```python
from build123d import *

# Parameters (mm, degrees)
F0_R         = 38.1
F1_DEPTH     = 381
F2_R         = 25.4
F3_DEPTH     = 304.8
F4_W         = 38.1
F4_H         = 63.5
F5_DEPTH     = 12.7
F7_DEPTH     = 203.2
F8_R         = 38.09999
F9_T3_ANGLE  = 359.64
F9_S4_R      = 38.1
F9_T5_DEPTH  = 21
F9_T8_ANGLE  = 230.2151920397
F9_S9_R      = 38.1
F9_T10_DEPTH = 20
F10_W        = 50.8
F10_H        = 12.7
F11_DEPTH    = 25.4
F13_DEPTH    = 12.7
F15_D        = 25.4
F16_W        = 25.4
F16_H        = 12.7
F17_DEPTH    = 12.7
F19_DEPTH    = 12.7
F21_D        = 12.7


# Not quite as in the source:
# - a fillet or chamfer that OpenCascade refuses, or shapes differently, is made with other operations: its cross-section is extruded or revolved along the edge and cut away or added
# - a fillet or chamfer is up to 0.001 mm smaller than in the source, because OpenCascade refuses the exact size


with BuildPart() as f1:
    # F0 (on Top) → F1 (new body)
    with BuildSketch(Plane.XY):
        Circle(F0_R)
    extrude(amount=F1_DEPTH)

    # F2 (on Top) → F3 (join)
    with BuildSketch(Plane.XY):
        Circle(F2_R)
    extrude(amount=-F3_DEPTH)

    # F4 (on Top) → F5 (join)
    with BuildSketch(Plane.XY):
        with Locations((19.05, 31.75)):
            Rectangle(F4_W, F4_H)
        with Locations((-19.05, 31.75)):
            Rectangle(F4_W, F4_H)
    extrude(amount=F5_DEPTH)

    # F6 (on face) → F7 (join)
    with BuildSketch(Plane.XY.offset(12.7)):
        with BuildLine():
            ThreePointArc((0.6819155813, 38.0938970327), (9.2181974345, 42.0397400715), (12.7, 50.7755763829))
            ThreePointArc((12.7, 50.7755763829), (-8.7358363114, 59.9937738174), (-0.6819155813, 38.0938970327))
            ThreePointArc((-0.6819155813, 38.0938970327), (0, 38.1), (0.6819155813, 38.0938970327))
        make_face()
        with BuildLine():
            ThreePointArc((0.6819155813, 38.0938970327), (0, 38.1), (-0.6819155813, 38.0938970327))
            ThreePointArc((-0.6819155813, 38.0938970327), (0, 38.0755763829), (0.6819155813, 38.0938970327))
        make_face()
    extrude(amount=F7_DEPTH)

    # F8 (radius 38.1 in the source; OpenCascade refuses exactly that, so slightly less here)
    f8_edges = [f1.edges().sort_by_distance(p)[0] for p in [
        (-38.1, 63.5, 6.35),
        (38.1, 63.5, 6.35),
    ]]
    fillet(f8_edges, radius=F8_R)

    # F9: fillet of radius 12.7 on 2 edges, made by hand


with BuildPart() as f9_tool1:
    # F9_s2 → F9_t3 (revolve)
    with BuildSketch(Plane.XZ.offset(-50.7755763829)):
        with BuildLine():
            ThreePointArc((0, 215.9), (8.9802561211, 212.1802561211), (12.7, 203.2))
            Line((12.7, 203.2), (12.7, 215.9))
            Line((12.7, 215.9), (0, 215.9))
        make_face()
    revolve(axis=Axis((0, 50.7755763829, 215.9), (0, 0, 1)), revolution_arc=F9_T3_ANGLE)

    # F9_s4 → F9_t5 (cut, symmetric)
    with BuildSketch(Plane.XY.offset(209.5)):
        Circle(F9_S4_R)
    extrude(amount=F9_T5_DEPTH, both=True, mode=Mode.SUBTRACT)


with BuildPart() as f9_tool6:
    # F9_s7 → F9_t8 (revolve)
    with BuildSketch(Plane(origin=(24.9682702957, 20.7915649924, 0), x_dir=(0, 0, 1), z_dir=(0.7684532224, 0.6399059658, 0))):
        with BuildLine():
            ThreePointArc((203.2, -51.7186552898), (212.1802561211, -47.9989114109), (215.9, -39.0186552898))
            Line((215.9, -39.0186552898), (215.9, -51.7186552898))
            Line((215.9, -51.7186552898), (203.2, -51.7186552898))
        make_face()
    revolve(axis=Axis((0, 50.7755763829, 215.9), (0, 0, 1)), revolution_arc=F9_T8_ANGLE)

    # F9_s9 → F9_t10 (cut, symmetric)
    with BuildSketch(Plane.XY.offset(209.5)):
        Circle(F9_S9_R)
    extrude(amount=F9_T10_DEPTH, both=True, mode=Mode.SUBTRACT)


with BuildPart() as f1_1:
    add(f1.part)

    # F9_t11: cut F9_tool1, F9_tool6
    add([f9_tool1.part, f9_tool6.part], mode=Mode.SUBTRACT)

    # F10 (on face) → F11 (join)
    with BuildSketch(Plane.XY.offset(381)):
        Rectangle(F10_W, F10_H)
    extrude(amount=F11_DEPTH)

    # F12 (on face) → F13 (join)
    with BuildSketch(Plane(origin=(0, 6.35, 0), x_dir=(-1, 0, 0), z_dir=(0, 1, 0))):
        with BuildLine():
            Line((-25.4, 406.4), (25.4, 406.4))
            ThreePointArc((25.4, 406.4), (0, 431.8), (-25.4, 406.4))
        make_face()
    extrude(amount=-F13_DEPTH)

    # F15 (through all)
    with Locations(Plane(origin=(0, 6.35, 0), x_dir=(-1, 0, 0), z_dir=(0, 1, 0))):
        with Locations((0, 406.4)):
            Hole(F15_D / 2)

    # F16 (on face) → F17 (join)
    with BuildSketch(Plane(origin=(0, 0, -304.8), x_dir=(1, 0, 0), z_dir=(0, 0, -1))):
        Rectangle(F16_W, F16_H)
    extrude(amount=F17_DEPTH)

    # F18 (on face) → F19 (join)
    with BuildSketch(Plane.XZ.offset(6.35)):
        with BuildLine():
            Line((12.7, -317.5), (-12.7, -317.5))
            ThreePointArc((-12.7, -317.5), (0, -330.2), (12.7, -317.5))
        make_face()
    extrude(amount=-F19_DEPTH)

    # F21 (through all)
    with Locations(Plane.XZ.offset(6.35)):
        with Locations((0, -317.5)):
            Hole(F21_D / 2)


solid = f1_1.part
```
Geometry check sheet. Reference: the model listing, model coordinates, mm. A direction names the side the tool comes from. Give positions to 0.01 mm unless a question says otherwise; leave off trailing zeros. Loops run counter-clockwise (first coordinate to the right, second up) from the corner with the lowest first, then second, coordinate; pieces in that order, holes last. Notation, with made-up numbers: M 42.5,-24.5 L 80.5,-24.5 A9 cw 80.5,-12.5 Z; hole C 22.25,52 d11. An arc over 180 degrees is marked long. Write item = value, one per line. Start each with the question number.
1. Tool access check on faces 1 (the face through (-12.7, 0, -311)), 2 (the face through (12.7, 0, -311)), 3 (the face through (-25.4, 0, 394)), 4 (the face through (-9, 25, 0)). Record the directions out of +Z, -Z, +X, -X, +Y, -Y that give a thin tool (end or side, any length) a straight path to the whole face; none if there is none.
2. Thickness scan on probe 1 along Z at (x, y) = (0, -2); probe 2 along X at (y, z) = (2, 406); probe 3 along Z at (x, y) = (-28.5, 37). Record the ranges inside material, lowest first.
3. Section check B-B, the plane z = -243. Enter the section's corners in (x, y).
4. Section check A-A, the plane z = 73. Enter the section's corners in (x, y).
5. Go/stop test with flat-tipped pins: P1, Ø23, axis at x = 0, z = 406.4, coming from the -Y side; P2, Ø8, axis at y = 24.5, z = 124.5, coming from the -X side; P3, Ø6, axis at y = 1.5, z = -79, coming from the -X side; P4, Ø3, axis at x = -20.5, z = 63, coming from the +Y side. Record where each tip stops, or that it passes through.
Values follow:
q1.face_1 = -Z, -X, +Y, -Y
q1.face_2 = -Z, +X, +Y, -Y
q1.face_3 = +Z, -X, +Y, -Y
q1.face_4 = -Z
q2.probe_1 = -330.2 to -323.85, -311.15 to 393.7, 419.1 to 431.8
q2.probe_2 = -25.4 to -12.69, 12.69 to 25.4
q2.probe_3 = 0 to 12.7
q3.outline = C 0,0 d50.8
q4.outline = M -0.68,38.09 A38.1 ccw long 0.68,38.09 A12.7 ccw long Z
q5.P1 = through
q5.P2 = -32.11
q5.P3 = -25.4
q5.P4 = 33.02
